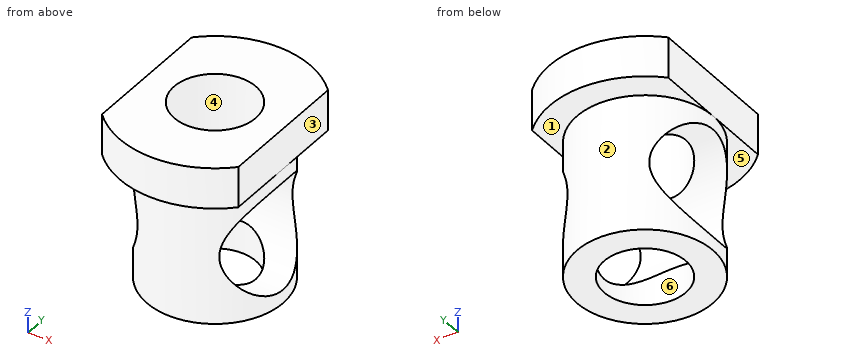
from build123d import *

# Parameters (mm, degrees)
SKETCH_1_R          = 2.5
EXTRUDE_1_DEPTH     = 5
EXTRUDE_2_DEPTH     = 1.5
SKETCH_3_R          = 1.5
CUT_EXTRUDE_1_DEPTH = 7.5
SKETCH_4_R          = 2
CUT_EXTRUDE_2_DEPTH = 5


with BuildPart() as part:
    # 草图1 → 凸台-拉伸1 (new body)
    with BuildSketch(Plane.XY):
        Circle(SKETCH_1_R)
    extrude(amount=EXTRUDE_1_DEPTH)

    # 草图2 → 凸台-拉伸2 (add)
    with BuildSketch(Plane.XY.offset(5)):
        with BuildLine():
            Line((-2.5, 2.449489743), (-2.5, -2.449489743))
            ThreePointArc((-2.5, -2.449489743), (0, -3.5), (2.5, -2.449489743))
            Line((2.5, -2.449489743), (2.5, 2.449489743))
            ThreePointArc((2.5, 2.449489743), (0, 3.5), (-2.5, 2.449489743))
        make_face()
    extrude(amount=EXTRUDE_2_DEPTH)

    # 草图3 → 切除-拉伸1 (cut, through all)
    with BuildSketch(Plane.XY.offset(6.5)):
        Circle(SKETCH_3_R)
    extrude(amount=-CUT_EXTRUDE_1_DEPTH, mode=Mode.SUBTRACT)

    # 草图4 → 切除-拉伸2 (cut, symmetric)
    with BuildSketch(Plane(origin=(0, 0, 0), x_dir=(0, 0, -1), z_dir=(1, 0, 0))):
        with Locations((-2.5, 0)):
            Circle(SKETCH_4_R)
    extrude(amount=CUT_EXTRUDE_2_DEPTH, both=True, mode=Mode.SUBTRACT)


solid = part.part
Design review of the part built by this model. Coordinates are the model's own, in mm. Face numbers are marked on the shaded views. A direction names the side the tool comes from. Give positions to 0.01 mm unless a question says otherwise; leave off trailing zeros. Order: outer loops, then holes, each group sorted by start corner. A loop starts at its lowest first (then second) coordinate and runs counter-clockwise, first axis right, second up.
1. To check wall thickness, follow L1, parallel to Y at x = 0, z = 0.9; L2, parallel to X at y = 2, z = 3.5. State the ranges of each line that lie inside material, in increasing order.
Solution:
L1: y = -2.5 to -1.5, 1.5 to 2.5
L2: x = -1.5 to 1.5
2. Add section A-A, the plane x = 0. State the section outline as (y, z) points, then the cut area to 3 significant figures.
Solution:
outline: (-3.5, 5) - (-2.5, 5) - (-2.5, 0) - (-1.5, 0) - (-1.5, 1.18) arc R2 cw to (-1.5, 3.82) - (-1.5, 6.5) - (-3.5, 6.5) - close; (1.5, 0) - (2.5, 0) - (2.5, 5) - (3.5, 5) - (3.5, 6.5) - (1.5, 6.5) - (1.5, 3.82) arc R2 cw to (1.5, 1.18) - close
area: 14.2 mm2
3. Mouldability with a two-part tool opening along X and no side actions: class the marked faces 1, 2, 3 and 4 as +X half, -X half, draft (parallel to the pull), parting line (faces both ways), or undercut.
Solution:
face 1: draft
face 2: parting line
face 3: +X half
face 4: undercut
4. Tool access review of the marked faces 5 and 6: name each direction out of +Z, -Z, +X, -X, +Y, -Y from which nothing blocks a thin tool from reaching the whole face with its end or side.
Solution:
face 5: -Z, -Y
face 6: +Z, -Z
5. Add section C-C, the plane z = 0.75. State the section outline as (x, y) points, then the cut area to 3 significant figures.
Solution:
outline: (-2.3, -0.97) arc R2.5 ccw to (2.3, -0.97) - (1.15, -0.97) arc R1.5 cw to (-1.15, -0.97) - close; (-2.3, 0.97) - (-1.15, 0.97) arc R1.5 cw to (1.15, 0.97) - (2.3, 0.97) arc R2.5 ccw to start
area: 8.51 mm2
6. Add section B-B, the plane y = -0.75. State the section outline as (x, z) points, then the cut area to 3 significant figures.
Solution:
outline: (-2.5, 5) - (-2.38, 5) - (-2.38, 4.35) - (-1.3, 4.35) - (-1.3, 6.5) - (-2.5, 6.5) - close; (-2.38, 0) - (-1.3, 0) - (-1.3, 0.65) - (-2.38, 0.65) - close; (1.3, 0) - (2.38, 0) - (2.38, 0.65) - (1.3, 0.65) - close; (1.3, 4.35) - (2.38, 4.35) - (2.38, 5) - (2.5, 5) - (2.5, 6.5) - (1.3, 6.5) - close
area: 6.41 mm2
7. Add section D-D, the plane x = -1.85. State the section outline as (y, z) points.
Solution:
outline: (-2.97, 5) - (-1.68, 5) - (-1.68, 3.58) arc R2 cw to (1.68, 3.58) - (1.68, 5) - (2.97, 5) - (2.97, 6.5) - (-2.97, 6.5) - close; (-1.68, 0) - (1.68, 0) - (1.68, 1.42) arc R2 cw to (-1.68, 1.42) - close
8. For pin 1 Ø1 at (x, z) = (0, 3.5) entering from -Y; pin 2 Ø2.5 at (x, y) = (0, 0) entering from +Z; pin 3 Ø2 at (y, z) = (1, 4.5) entering from -X; pin 4 Ø2 at (y, z) = (-2.5, 1.5) entering from +X, all flat-tipped, find the tip position at first contact; note any pin that passes through.
Solution:
pin 1: stops at y = -2.5
pin 2: passes through
pin 3: stops at x = -2.5
pin 4: stops at x = 1.97
